```python
from build123d import *

# Parameters (mm, degrees)
SKETCH23_R               = 24
SKETCH23_R_2             = 17.5
BOSS_EXTRUDE3_DEPTH      = 2
MOVE_FACE1_BY            = 0.15
CHAMFER2_SIZE            = 0.5
CUT_EXTRUDE3_DEPTH       = 2
FILLET1_R                = 0.5
CIRPATTERN1_COUNT        = 3
FILLET1_OF_CIRPATTERN1_R = 0.5


with BuildPart() as part:
    # Sketch23 → Boss-Extrude3 (new body)
    with BuildSketch(Plane(origin=(0, 0, 0), x_dir=(-1, 0, 0), z_dir=(0, 0, -1))):
        Circle(SKETCH23_R)
        Circle(SKETCH23_R_2, mode=Mode.SUBTRACT)
    extrude(amount=-BOSS_EXTRUDE3_DEPTH)

    # Move Face1: a curved face moved inward by 0.15
    add(Solid.thicken(part.faces().sort_by_distance((17.5, 0, 1))[0], -MOVE_FACE1_BY), mode=Mode.SUBTRACT)

    # Chamfer2
    chamfer2_edges = [part.edges().sort_by_distance(p)[0] for p in [
        (24, 0, 0),
        (24, 0, 2),
        (17.65, 0, 2),
        (17.65, 0, 0),
    ]]
    chamfer(chamfer2_edges, length=CHAMFER2_SIZE)

    # Sketch24 → Cut-Extrude3 (cut)
    with BuildSketch(Plane(origin=(0, 0, 0), x_dir=(-1, 0, 0), z_dir=(0, 0, -1))):
        with BuildLine():
            Line((-5, 20.396078054), (-5, 16.926975512))
            ThreePointArc((-5, 16.926975512), (0, 17.65), (5, 16.926975512))
            Line((5, 16.926975512), (5, 20.396078054))
            ThreePointArc((5, 20.396078054), (0, 21), (-5, 20.396078054))
        make_face()
    cut_extrude3 = extrude(amount=-CUT_EXTRUDE3_DEPTH, mode=Mode.SUBTRACT)

    # Fillet1
    fillet1_edges = [part.edges().sort_by_distance(p)[0] for p in [
        (5, 20.396078054, 1),
        (-5, 20.396078054, 1),
    ]]
    fillet(fillet1_edges, radius=FILLET1_R)

    # CirPattern1: Cut-Extrude3 ×3 about axis
    cirpattern1_axis = Axis((0, 0, 0), (0, 0, 1))
    for i in range(1, CIRPATTERN1_COUNT):
        add(cut_extrude3.rotate(cirpattern1_axis, i * 360 / CIRPATTERN1_COUNT), mode=Mode.SUBTRACT)

    # Fillet1 of CirPattern1
    fillet1_of_cirpattern1_edges = [part.edges().sort_by_distance(p)[0] for p in [
        (-20.163521733, -5.867912008, 1),
        (-15.163521733, -14.528166046, 1),
        (15.163521733, -14.528166046, 1),
        (20.163521733, -5.867912008, 1),
    ]]
    fillet(fillet1_of_cirpattern1_edges, radius=FILLET1_OF_CIRPATTERN1_R)


solid = part.part
```
For this review, take the finished solid that the model builds, in its own axes (mm). A direction names the side the tool comes from. Give positions to 0.01 mm unless a question says otherwise; leave off trailing zeros. Write each loop counter-clockwise with the first axis right and the second up, starting at its lowest first coordinate (ties: lowest second). Pieces come first, ordered by that corner, then holes. Notation, with made-up numbers: M 36.5,-11 L 59.5,-11 A10 ccw 59.5,-7 Z; hole C -31.75,-32.75 d11. An arc over 180 degrees is marked long. Answer as CSV lines item,"result".
1. For pin 1 (8 mm diameter, centred on x = -11, y = 10, fed in from -Z); pin 2 (1 mm diameter, centred on y = 3.5, z = 1, fed in from -X); pin 3 (1 mm diameter, centred on x = -7, z = 0.5, fed in from +Y); pin 4 (0.6 mm diameter, centred on y = 18.5, z = 1, fed in from +X), all flat-tipped, find the tip position at first contact; note any pin that passes through.
Findings:
pin 1,"stops at z = 0"
pin 2,"stops at x = -23.81"
pin 3,"stops at y = 23.1"
pin 4,"stops at x = 15.64"
2. Consider section B-B, the plane y = 0. Write out the cut boundary in (x, z).
Findings:
outline,"M -24,0.5 L -23.5,0 L -18.15,0 L -17.65,0.5 L -17.65,1.5 L -18.15,2 L -23.5,2 L -24,1.5 Z; M 17.65,0.5 L 18.15,0 L 23.5,0 L 24,0.5 L 24,1.5 L 23.5,2 L 18.15,2 L 17.65,1.5 Z"
3. For faces 4 (the flat face through (-12, -14, 2)), 5 (the conical face through (0.191, -17.784, 1.635)), 6 (the flat face through (-18.508, -4.912, 0.986)), 7 (the conical face through (-15.5, 8.73, 0.36)), list the 3-axis set-ups (+Z, -Z, +X, -X, +Y, -Y) from which the entire face can be reached by the end or side of a thin tool; tool diameter is ignored.
Findings:
face 4,"+Z, +X, -X, +Y, -Y"
face 5,"+Z"
face 6,"+Z, -Z"
face 7,"-Z"
4. Wall thickness on line 1 (Y direction, x = 0, z = 1.4); line 2 (X direction, y = -14, z = 1.9); line 3 (Y direction, x = 3, z = 1.05): over which ranges is each line inside the solid? List them lowest first.
Findings:
line 1,"y = -24 to -17.65, 21 to 24"
line 2,"x = -19 to -15.65, -14.25 to -11.39, 11.39 to 14.25, 15.65 to 19"
line 3,"y = -23.81 to -17.39, 20.78 to 23.81"
5. Consider section A-A, the plane x = 0. Write out the cut boundary in (y, z), then the cut area to 4 significant figures.
Findings:
outline,"M -24,0.5 L -23.5,0 L -18.15,0 L -17.65,0.5 L -17.65,1.5 L -18.15,2 L -23.5,2 L -24,1.5 Z; M 21,0 L 23.5,0 L 24,0.5 L 24,1.5 L 23.5,2 L 21,2 Z"
area,"17.95 mm2"
6. Draft analysis for pull direction Y (two halves, no side actions). For faces 1 (the flat face through (13.508, -13.573, 0.986)), 2 (the cylindrical face through (23.977, 1.055, 0.993)), 3 (the flat face through (-12, -14, 0)), state which applies: +Y half, -Y half, draft (parallel to the pull), parting line (faces both ways), or undercut.
Findings:
face 1,"undercut"
face 2,"parting line"
face 3,"draft"
